Check sheet for the drawn part. Datum: minimum x, y, z corner. Units: mm. A direction names the side the tool comes from. Give positions to 0.01 mm unless a question says otherwise; leave off trailing zeros. Loops run counter-clockwise (first coordinate to the right, second up) from the corner with the lowest first, then second, coordinate; pieces in that order, holes last.
1. Cross-section at B-B, the plane x = 7. Record the cut outline in (y, z), plus the area to 3 significant figures.
2. Tool access check on the marked faces 1 and 2. Record the directions out of +Z, -Z, +X, -X, +Y, -Y that give a thin tool (end or side, any length) a straight path to the whole face; none if there is none.
3. Go/stop test with flat-tipped pins: pin 1 Ø1 at (y, z) = (9.5, 8) entering from -X; pin 2 Ø1.4 at (y, z) = (7.5, 26) entering from -X; pin 3 Ø2 at (x, y) = (12.5, 12.5) entering from +Z. Record where each tip stops, or that it passes through.
4. Release check for a two-part mould opening along X. For the marked faces 3, 4 and 5 record: +X half, -X half, draft (parallel to the pull), parting line (faces both ways), or undercut.
5. Material ranges on L1, parallel to Z at x = 6.5, y = 2; L2, parallel to Z at x = 12, y = 10; L3, parallel to X at y = 12.25, z = 12.75 (1 decimal), recorded low to high.
6. Cross-section at C-C, the plane z = 13.75. Record the cut outline in (x, y).
7. Cross-section at A-A, the plane y = 7. State how many separate pieces and enclosed holes the cut face has, plus the area to 3 significant figures.
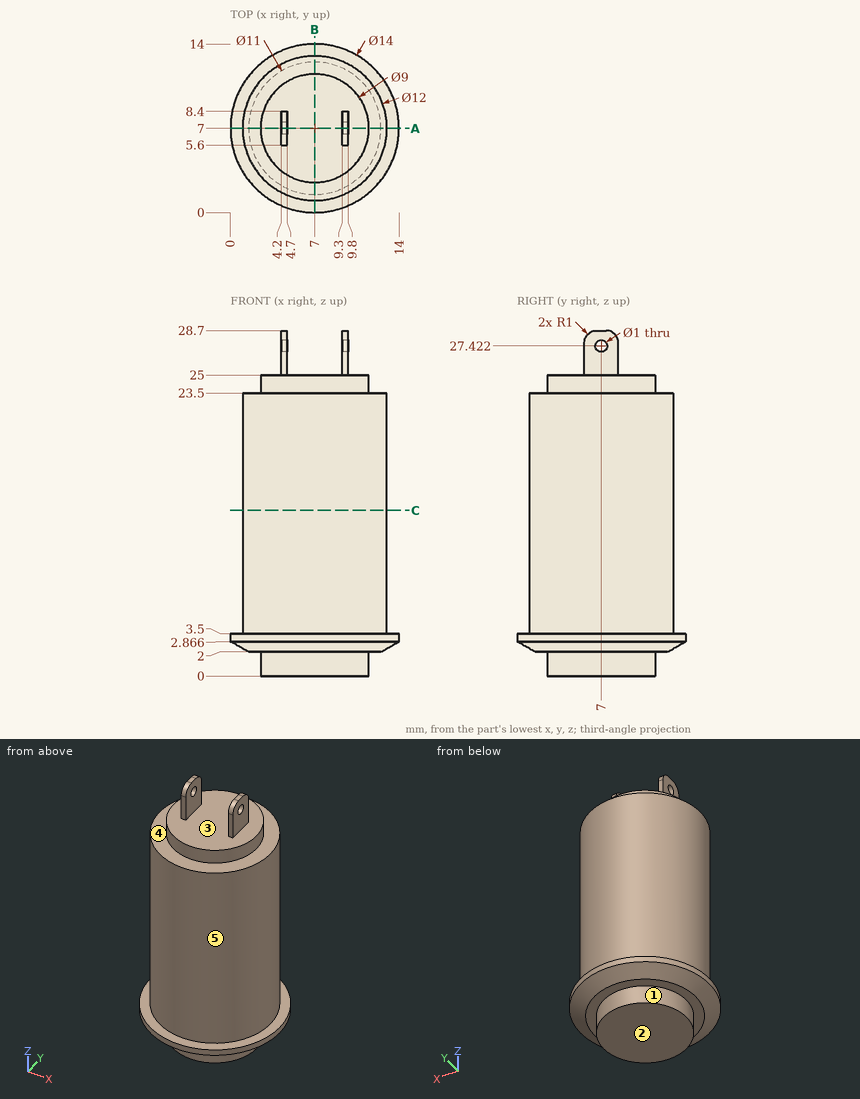
Result:
1. outline: (0, 2.87) - (1.5, 2) - (2.5, 2) - (2.5, 0) - (11.5, 0) - (11.5, 2) - (12.5, 2) - (14, 2.87) - (14, 3.5) - (13, 3.5) - (13, 23.5) - (11.5, 23.5) - (11.5, 25) - (2.5, 25) - (2.5, 23.5) - (1, 23.5) - (1, 3.5) - (0, 3.5) - close
1. area: 291 mm2
2. face 1: -Z
2. face 2: -Z, +X, -X, +Y, -Y
3. pin 1: stops at x = 1.34
3. pin 2: stops at x = 4.2
3. pin 3: stops at z = 3.5
4. face 3: undercut
4. face 4: draft
4. face 5: parting line
5. L1: z = 2 to 23.5
5. L2: z = 2.19 to 23.5
5. L3: x = 4.1 to 9.9
6. outline: circle Ø12 at (7, 7)
7. separate pieces: 3
7. enclosed holes: 0
7. area: 294 mm2
